Here's how the part is built. I have some questions about the finished solid (model axes, mm). Coordinates: 2 decimals unless noted, no trailing zeros. Loops run counter-clockwise (first coordinate to the right, second up) from the corner with the lowest first, then second, coordinate; pieces in that order, holes last.
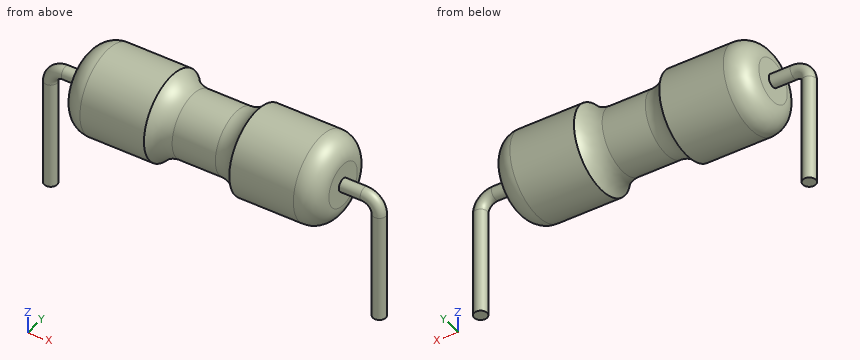
from build123d import *

# Parameters (mm, degrees)
SKETCH_2_R = 0.15


with BuildPart() as part:
    # 草图1 → 旋转1 (revolve)
    with BuildSketch(Plane.XY, mode=Mode.PRIVATE) as revolve_1_sk:
        with BuildLine():
            Line((3, 0.5), (3, 0))
            Line((3, 0), (-3, 0))
            Line((-3, 0), (-3, 0.5))
            ThreePointArc((-3, 0.5), (-2.853553391, 0.853553391), (-2.5, 1))
            Line((-2.5, 1), (-1, 1))
            ThreePointArc((-1, 1), (-0.780842208, 0.819581425), (-0.505634241, 0.75))
            Line((-0.505634241, 0.75), (0.505634241, 0.75))
            ThreePointArc((0.505634241, 0.75), (0.780842208, 0.819581425), (1, 1))
            Line((1, 1), (2.5, 1))
            ThreePointArc((2.5, 1), (2.853553391, 0.853553391), (3, 0.5))
        make_face()
    revolve(revolve_1_sk.sketch.rotate(Axis((-1000, 0, 0), (1, 0, 0)), 90), axis=Axis((-1000, 0, 0), (1, 0, 0)))

    # 扫描1: sweep along a path in 草图3
    with BuildLine(Plane(origin=(0, 0, 0), x_dir=(1, 0, 0), z_dir=(0, 1, 0))) as sweep_1_path:
        Line((3, -0.15), (3.5, -0.15))
        ThreePointArc((3.5, -0.15), (3.853553391, -0.003553391), (4, 0.35))
        Line((4, 0.35), (4, 2.85))
    # 草图2 → 扫描1 (sweep)
    with BuildSketch(Plane(origin=(3, 0, 0), x_dir=(0, 0, -1), z_dir=(1, 0, 0))):
        Circle(SKETCH_2_R)
    sweep_1 = sweep(path=sweep_1_path.line)

    # 镜向1: 扫描1 across plane
    add(sweep_1.mirror(Plane(origin=(0, 0, 0), x_dir=(0, 0, 1), z_dir=(1, 0, 0))))


solid = part.part
Q1. Suppose I cut it at A-A on z = -1.7. Write out the boundary of the cut face in (x, y).
Q2. Suppose I cut it at D-D on x = -1.75. Write out the boundary of the cut face in (y, z), and give its area (3 significant figures).
Q3. Suppose I cut it at C-C on x = 0. Write out the boundary of the cut face in (y, z), and give its area (3 significant figures).
Q4. Will this pin go through, and if not, where does the flat tip stop? P1, Ø1.5, axis at x = 0, z = 0.5, coming from the +Y side.
Q5. Please list where these lines run through material, in increasing order: probe 1 along X at (y, z) = (-0.05, -0.25); probe 2 along X at (y, z) = (-0.4, -0.1); probe 3 along Z at (x, y) = (-1.75, 0.25).
Check values:
1. outline: circle Ø0.3 at (-3.85, 0); circle Ø0.3 at (3.85, 0)
2. outline: circle Ø2 at (0, 0)
2. area: 3.14 mm2
3. outline: circle Ø1.5 at (0, 0)
3. area: 1.77 mm2
4. P1: stops at y = 0.76
5. probe 1: x = -3.98 to -3.68, -3 to 3, 3.68 to 3.98
5. probe 2: x = -3 to 3
5. probe 3: z = -0.97 to 0.97
